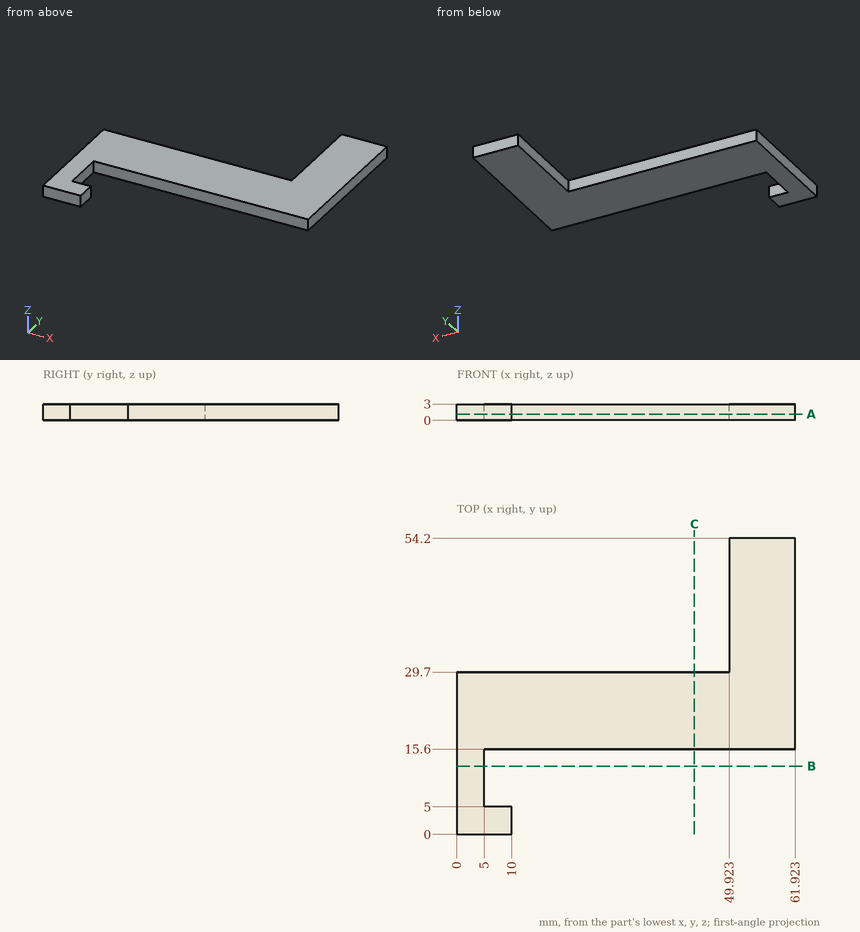
Drawing for the job (mm, zero at the part's lowest x, y, z). Give positions to 0.01 mm unless a question says otherwise; leave off trailing zeros. Write each loop counter-clockwise with the first axis right and the second up, starting at its lowest first coordinate (ties: lowest second). Pieces come first, ordered by that corner, then holes. Notation, with made-up numbers: (74.5, 76) - (111.5, 76) arc R17 ccw to (111.5, 94) - close; hole circle Ø8 at (-32, 29). An arc over 180 degrees is marked (long way). Answer as CSV lines item,"result".
Q1. Flat gauge pins, fed straight in: pin 1 Ø0.9 at (x, z) = (32.5, 2) entering from -Y; pin 2 Ø1.5 at (x, z) = (22.5, 1.5) entering from +Y; pin 3 Ø1.5 at (y, z) = (12, 2) entering from +X. Where does each tip first touch, or does it go through?
Result set:
pin 1,"y = 15.6"
pin 2,"y = 29.7"
pin 3,"x = 5"
Q2. Band-saw the part on A-A (z = 1.15). Give the cut face in (x, y), and give its area (3 significant figures).
Result set:
outline,"(0, 0) - (10, 0) - (10, 5) - (5, 5) - (5, 15.6) - (61.92, 15.6) - (61.92, 54.2) - (49.92, 54.2) - (49.92, 29.7) - (0, 29.7) - close"
area,"1,270 mm²"
Q3. Drill centre lines: line 1 (X direction, y = 15, z = 0.7); line 2 (X direction, y = 46, z = 1.8); line 3 (Y direction, x = 9, z = 0.85). Where is each one in solid material? Low to high. Write a range as from..to.
Result set:
line 1,"0..5"
line 2,"49.92..61.92"
line 3,"0..5, 15.6..29.7"
Q4. Band-saw the part on C-C (x = 43.5). Give the cut face in (y, z).
Result set:
outline,"(15.6, 0) - (29.7, 0) - (29.7, 3) - (15.6, 3) - close"
Q5. Band-saw the part on B-B (y = 12.5). Give the cut face in (x, z).
Result set:
outline,"(0, 0) - (5, 0) - (5, 3) - (0, 3) - close"
